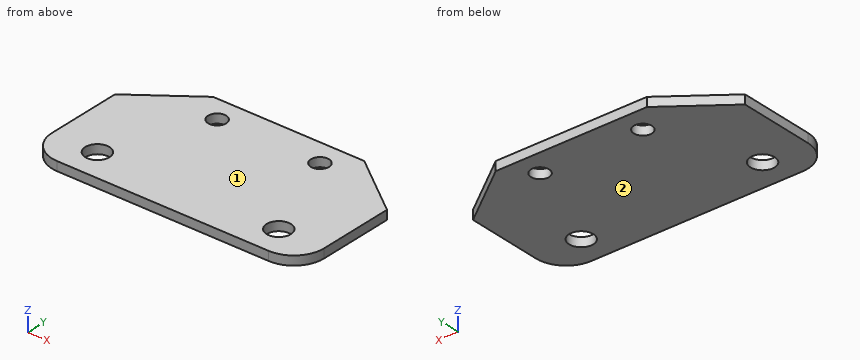
```python
from build123d import *

# Parameters (mm, degrees)
SKETCH1_R           = 3
SKETCH1_R_2         = 4
BOSS_EXTRUDE1_DEPTH = 3
FILLET1_R           = 10


with BuildPart() as part:
    # Sketch1 → Boss-Extrude1 (new body)
    with BuildSketch(Plane.XY):
        Polygon((0, 35), (20, 50), (70, 50), (90, 35), (90, 0), (0, 0), align=None)
        with Locations((28, 42)):
            Circle(SKETCH1_R, mode=Mode.SUBTRACT)
        with Locations((15, 10)):
            Circle(SKETCH1_R_2, mode=Mode.SUBTRACT)
        with Locations(Location((75, 10, 0), (0, 0, 180))):
            Circle(SKETCH1_R_2, mode=Mode.SUBTRACT)
        with Locations(Location((62, 42, 0), (0, 0, 180))):
            Circle(SKETCH1_R, mode=Mode.SUBTRACT)
    extrude(amount=BOSS_EXTRUDE1_DEPTH)

    # Fillet1
    fillet1_edges = [part.edges().sort_by_distance(p)[0] for p in [
        (90, 0, 1.5),
        (0, 0, 1.5),
    ]]
    fillet(fillet1_edges, radius=FILLET1_R)


solid = part.part
```
For this review, take the finished solid that the model builds, in its own axes (mm). Face numbers are marked on the shaded views. Give positions to 0.01 mm unless a question says otherwise; leave off trailing zeros. Write each loop counter-clockwise with the first axis right and the second up, starting at its lowest first coordinate (ties: lowest second). Pieces come first, ordered by that corner, then holes.
Item 1: The part is to be moulded in two halves that separate along Z. For the marked faces 1 and 2, say which applies: +Z half, -Z half, draft (parallel to the pull), parting line (faces both ways), or undercut.
Item 2: Take a section at B-B (z = 1.7). Give the boundary of the cut face in (x, y).
Item 3: Take a section at D-D (y = 7). Give the boundary of the cut face in (x, z), and give its area (3 significant figures).
Item 4: Wall thickness on probe 1 along Y at (x, z) = (62, 1.6); probe 2 along X at (y, z) = (40, 0.9); probe 3 along Y at (x, z) = (75, 2.05): over which ranges is each line inside the solid? List them lowest first.
Item 5: Insertion check: P1, Ø1.5, axis at y = 6.5, z = 0.5, coming from the -X side. The pin has a flat end and moves straight along its axis. Give the tip position at first contact, or say it passes through.
Item 6: Take a section at C-C (y = 42). Give the boundary of the cut face in (x, z).
Item 7: Take a section at A-A (x = 28). Give the boundary of the cut face in (y, z).
Established:
1. face 1: +Z half
1. face 2: -Z half
2. outline: (0, 10) arc R10 ccw to (10, 0) - (80, 0) arc R10 ccw to (90, 10) - (90, 35) - (70, 50) - (20, 50) - (0, 35) - close; hole circle Ø8 at (15, 10); hole circle Ø6 at (28, 42); hole circle Ø6 at (62, 42); hole circle Ø8 at (75, 10)
3. outline: (0.46, 0) - (12.35, 0) - (12.35, 3) - (0.46, 3) - close; (17.65, 0) - (72.35, 0) - (72.35, 3) - (17.65, 3) - close; (77.65, 0) - (89.54, 0) - (89.54, 3) - (77.65, 3) - close
3. area: 235 mm2
4. probe 1: y = 0 to 39, 45 to 50
4. probe 2: x = 6.67 to 25.76, 30.24 to 59.76, 64.24 to 83.33
4. probe 3: y = 0 to 6, 14 to 46.25
5. P1: stops at x = 0.39
6. outline: (9.33, 0) - (25, 0) - (25, 3) - (9.33, 3) - close; (31, 0) - (59, 0) - (59, 3) - (31, 3) - close; (65, 0) - (80.67, 0) - (80.67, 3) - (65, 3) - close
7. outline: (0, 0) - (39, 0) - (39, 3) - (0, 3) - close; (45, 0) - (50, 0) - (50, 3) - (45, 3) - close
